Input: part model. Units: mm. Frame: model coordinates. A direction names the side the tool comes from. Give positions to 0.01 mm unless a question says otherwise; leave off trailing zeros. Loops run counter-clockwise (first coordinate to the right, second up) from the corner with the lowest first, then second, coordinate; pieces in that order, holes last.
from build123d import *

# Parameters (mm, degrees)
SKETCH1_W           = 27.8
SKETCH1_H           = 28
SKETCH1_R           = 2.55
BOSS_EXTRUDE1_DEPTH = 3.5
SKETCH2_W           = 27.8
SKETCH2_H           = 15.9
SKETCH2_R           = 1.55
BOSS_EXTRUDE2_DEPTH = 3
SKETCH3_W           = 6
SKETCH3_H           = 6
CUT_EXTRUDE5_DEPTH  = 3.5
SKETCH4_W           = 6
SKETCH4_H           = 6
SKETCH4_H_2         = 1
CUT_EXTRUDE7_DEPTH  = 3.5
SKETCH5_R           = 2.55
SKETCH5_R_2         = 5
CUT_EXTRUDE8_DEPTH  = 3


with BuildPart() as part:
    # Sketch1 → Boss-Extrude1 (new body)
    with BuildSketch(Plane(origin=(0, 0, 0), x_dir=(1, 0, 0), z_dir=(0, 1, 0))):
        with Locations((13.9, 14)):
            Rectangle(SKETCH1_W, SKETCH1_H)
        with Locations(Location((13.65, 23.68, 0), (0, 0, 270))):
            Circle(SKETCH1_R, mode=Mode.SUBTRACT)
        with Locations(Location((3.65, 23.68, 0), (0, 0, 270))):
            Circle(SKETCH1_R, mode=Mode.SUBTRACT)
    extrude(amount=BOSS_EXTRUDE1_DEPTH)

    # Sketch2 → Boss-Extrude2 (add)
    with BuildSketch(Plane(origin=(0, 3.5, 0), x_dir=(1, 0, 0), z_dir=(0, 1, 0))):
        with Locations((13.9, 7.95)):
            Rectangle(SKETCH2_W, SKETCH2_H)
        with Locations(Location((2.8, 2.8, 0), (0, 0, 270))):
            Circle(SKETCH2_R, mode=Mode.SUBTRACT)
        with Locations(Location((25, 13.1, 0), (0, 0, 270))):
            Circle(SKETCH2_R, mode=Mode.SUBTRACT)
    extrude(amount=BOSS_EXTRUDE2_DEPTH)

    # Sketch3 → Cut-Extrude5 (cut)
    with BuildSketch(Plane.XZ):
        with Locations((3, -3)):
            Rectangle(SKETCH3_W, SKETCH3_H)
    extrude(amount=-CUT_EXTRUDE5_DEPTH, mode=Mode.SUBTRACT)

    # Sketch4 → Cut-Extrude7 (cut)
    with BuildSketch(Plane.XZ):
        with Locations((24.8, -12.9)):
            Rectangle(SKETCH4_W, SKETCH4_H)
        with Locations((24.8, -16.4)):
            Rectangle(SKETCH4_W, SKETCH4_H_2)
    extrude(amount=-CUT_EXTRUDE7_DEPTH, mode=Mode.SUBTRACT)

    # Sketch5 → Cut-Extrude8 (cut)
    with BuildSketch(Plane.XZ):
        with Locations(Location((13.65, -23.68, 0), (0, 0, 90))):
            Circle(SKETCH5_R)
        with Locations(Location((13.65, -13.68, 0), (0, 0, 270))):
            Circle(SKETCH5_R_2)
    extrude(amount=-CUT_EXTRUDE8_DEPTH, mode=Mode.SUBTRACT)


solid = part.part
(1) Cut plane C-C (y = 2.25). Return the cut outline in (x, z).
Values follow:
outline: (0, -28) - (27.8, -28) - (27.8, -16.9) - (21.8, -16.9) - (21.8, -9.9) - (27.8, -9.9) - (27.8, 0) - (6, 0) - (6, -6) - (0, -6) - close; hole circle Ø5.1 at (3.65, -23.68); hole circle Ø10 at (13.65, -13.68); hole circle Ø5.1 at (13.65, -23.68)
(2) Cut plane D-D (z = -2.8). Return the cut outline in (x, y).
Values follow:
outline: (0, 3.5) - (1.25, 3.5) - (1.25, 6.5) - (0, 6.5) - close; (4.35, 3.5) - (6, 3.5) - (6, 0) - (27.8, 0) - (27.8, 6.5) - (4.35, 6.5) - close
(3) Cut plane B-B (x = 13.65). Return the cut outline in (y, z), and give its area (4 significant figures).
Values follow:
outline: (0, -28) - (3.5, -28) - (3.5, -26.23) - (0, -26.23) - close; (0, -21.13) - (3.5, -21.13) - (3.5, -15.9) - (6.5, -15.9) - (6.5, 0) - (0, 0) - (0, -8.68) - (3, -8.68) - (3, -18.68) - (0, -18.68) - close
area: 97.85 mm2
(4) Pin query (flat end, axial travel): pin 1 Ø1.8 at (y, z) = (1.5, -14) entering from +X; pin 2 Ø5 at (x, z) = (25, -13.1) entering from -Y; pin 3 Ø6 at (x, z) = (13.65, -13.68) entering from -Y. Return the tip coordinate at first contact, or that it passes through.
Values follow:
pin 1: stops at x = 21.8
pin 2: stops at y = 3.5
pin 3: stops at y = 3
(5) Reachability of faces 4 (the flat face through (14, 3, -14)), 5 (the flat face through (14, 5, -15.9)), 6 (the flat face through (4.3, 3.5, -3.6)), 7 (the flat face through (25, 2, -9.9)) from +Z, -Z, +X, -X, +Y, -Y: full face, straight path, thin tool, end or side. Return the list, or none.
Values follow:
face 4: -Y
face 5: -Z, +X, -X, +Y
face 6: +Z, -X, -Y
face 7: +X, -Y
(6) Mould query, pull axis X, two halves, no side actions, for faces 1 (the flat face through (27.8, 3, -6)), 2 (the cylindrical face through (3.762, 1.726, -26.228)), 3 (the flat face through (20, 0, -14)). Classes: +X half, -X half, draft (parallel to the pull), parting line (faces both ways), or undercut.
Values follow:
face 1: +X half
face 2: undercut
face 3: draft
(7) Ray query, probe 1 along Z at (x, y) = (13.5, 1.25); probe 2 along X at (y, z) = (1.5, -23.68); probe 3 along Z at (x, y) = (14.25, 2.5). Return the intervals inside material, ascending.
Values follow:
probe 1: z = -28 to -26.23, -21.13 to -18.68, -8.68 to 0
probe 2: x = 0 to 1.1, 6.2 to 11.1, 16.2 to 27.8
probe 3: z = -28 to -26.16, -21.2 to -18.64, -8.72 to 0
(8) Cut plane A-A (z = -23.68). Return the cut outline in (x, y), and give its area (3 significant figures).
Values follow:
outline: (0, 0) - (1.1, 0) - (1.1, 3.5) - (0, 3.5) - close; (6.2, 0) - (11.1, 0) - (11.1, 3.5) - (6.2, 3.5) - close; (16.2, 0) - (27.8, 0) - (27.8, 3.5) - (16.2, 3.5) - close
area: 61.6 mm2
